Input: dimensioned drawing with shaded views. Units: mm. Origin: part minimum x, y, z. Give positions to 0.01 mm unless a question says otherwise; leave off trailing zeros. Write each loop counter-clockwise with the first axis right and the second up, starting at its lowest first coordinate (ties: lowest second). Pieces come first, ordered by that corner, then holes.
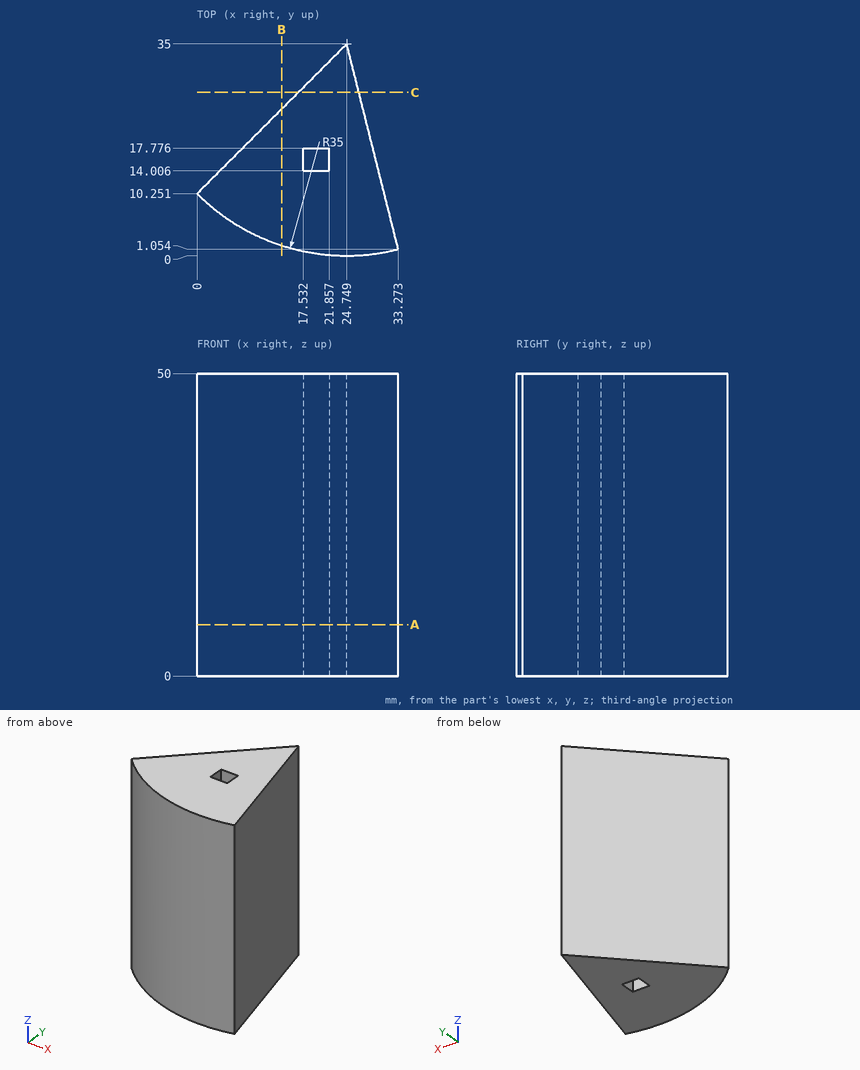
Item 1: Line query: L1, parallel to X at y = 8.5, z = 32.5 (1 decimal); L2, parallel to Y at x = 13, z = 30; L3, parallel to Y at x = 17, z = 41. Output: solid intervals per line, ascending.
Found:
L1: x = 1.9 to 31.4
L2: y = 2.03 to 23.25
L3: y = 0.87 to 27.25
Item 2: Section C-C, the plane y = 27. Return the cut outline in (x, z).
Found:
outline: (16.75, 0) - (26.76, 0) - (26.76, 50) - (16.75, 50) - close
Item 3: Section A-A, the plane z = 8.5. Return the cut outline in (x, y).
Found:
outline: (0, 10.25) arc R35 ccw to (33.27, 1.05) - (24.75, 35) - close; hole (17.53, 14.01) - (21.86, 14.01) - (21.86, 17.78) - (17.53, 17.78) - close
Item 4: Section B-B, the plane x = 14. Return the cut outline in (y, z).
Found:
outline: (1.69, 0) - (24.25, 0) - (24.25, 50) - (1.69, 50) - close
Item 5: Pin query (flat end, axial travel): pin 1 Ø1.9 at (y, z) = (17, 36) entering from -X; pin 2 Ø6 at (x, y) = (20.5, 4.5) entering from -Z; pin 3 Ø3 at (x, z) = (5, 25.5) entering from +Y; pin 4 Ø5 at (x, z) = (20.5, 17) entering from +Y. Return the tip coordinate at first contact, or that it passes through.
Found:
pin 1: stops at x = 5.8
pin 2: stops at z = 0
pin 3: stops at y = 16.75
pin 4: stops at y = 33.25
